Design review of the part built by this model. Coordinates are the model's own, in mm. Give positions to 0.01 mm unless a question says otherwise; leave off trailing zeros. Loops run counter-clockwise (first coordinate to the right, second up) from the corner with the lowest first, then second, coordinate; pieces in that order, holes last. Notation, with made-up numbers: M 89,-36 L 144,-36 A29 ccw 144,-8 Z; hole C 37,25 d5. An arc over 180 degrees is marked long. Use a Markdown table: item, result. Add a question column.
(1) Add section A-A, the plane y = 0. Give the boundary of the cut face in (x, z), then the cut area to 3 significant figures.
(2) Add section C-C, the plane z = -10. Give the boundary of the cut face in (x, y), then the cut area to 3 significant figures.
(3) For probe 1 along Z at (x, y) = (1.25, 0); probe 2 along Z at (x, y) = (1.55, -1.75); probe 3 along Y at (x, z) = (1.4, -16), list the stretches that pass through material, from the lowest coordinate up.
(4) Draft analysis for pull direction Y (two halves, no side actions). For faces 1 (the face through (1, 0, 19.5)), 2 (the face through (1, 0, 17)), 3 (the face through (0.9, -11, 0.3)), state which applies: pulls with the +Y half, pulls with the -Y half, needs draft (parallel to the pull), parting line crosses it, or undercut.
(5) Add section B-B, the plane z = -15. Give the boundary of the cut face in (x, y), then the cut area to 3 significant figures.
```python
from build123d import *

# Parameters (mm, degrees)
PAD011_DEPTH       = 19.5
SKETCH016_R        = 2
POCKET003_DEPTH    = 2.3
CHAMFER006_1_SIZE2 = 4
CHAMFER006_1_SIZE  = 1.5
CHAMFER006_2_SIZE2 = 4
CHAMFER006_2_SIZE  = 1.5
CHAMFER007_SIZE    = 0.2


with BuildPart() as part:
    # Sketch015 → Pad011 (new body, symmetric)
    with BuildSketch(Plane.XY):
        Polygon((0, -10.1), (0, 10.1), (1.8, 11.9), (2.3, 11.9), (2.3, -11.9), (1.8, -11.9), align=None)
    extrude(amount=PAD011_DEPTH, both=True)

    # Sketch016 (on Face4 of Pad011) → Pocket003 (cut)
    with BuildSketch(Plane.YZ.offset(2.3)):
        with Locations((0, 15)):
            Circle(SKETCH016_R)
        with Locations((0, -15)):
            Circle(SKETCH016_R)
    extrude(amount=-POCKET003_DEPTH, mode=Mode.SUBTRACT)

    # Chamfer006 1
    chamfer006_1_edges = [part.edges().sort_by_distance(p)[0] for p in [
        (2.05, -11.9, -19.5),
        (2.05, 11.9, -19.5),
    ]]
    chamfer006_1_side = part.faces().sort_by_distance((1.184602, 0, -19.5))[0]
    chamfer(chamfer006_1_edges, length=CHAMFER006_1_SIZE, length2=CHAMFER006_1_SIZE2, reference=chamfer006_1_side)

    # Chamfer006 2
    chamfer006_2_edges = [part.edges().sort_by_distance(p)[0] for p in [
        (2.05, -11.9, 19.5),
        (2.05, 11.9, 19.5),
    ]]
    chamfer006_2_side = part.faces().sort_by_distance((1.184602, 0, 19.5))[0]
    chamfer(chamfer006_2_edges, length=CHAMFER006_2_SIZE, length2=CHAMFER006_2_SIZE2, reference=chamfer006_2_side)

    # Chamfer007
    chamfer007_edges = [part.edges().sort_by_distance(p)[0] for p in [
        (2.3, -2, -15),
        (0, -2, -15),
        (2.3, -2, 15),
        (0, -2, 15),
    ]]
    chamfer(chamfer007_edges, length=CHAMFER007_SIZE)


solid = part.part
```
Established:
| question | item | result |
|---|---|---|
| 1 | outline | M 0,-19.5 L 2.3,-19.5 L 2.3,-17.2 L 2.1,-17 L 0.2,-17 L 0,-17.2 Z; M 0,-12.8 L 0.2,-13 L 2.1,-13 L 2.3,-12.8 L 2.3,12.8 L 2.1,13 L 0.2,13 L 0,12.8 Z; M 0,17.2 L 0.2,17 L 2.1,17 L 2.3,17.2 L 2.3,19.5 L 0,19.5 Z |
| 1 | area | 71.1 mm^2 |
| 2 | outline | M 0,-10.1 L 1.8,-11.9 L 2.3,-11.9 L 2.3,11.9 L 1.8,11.9 L 0,10.1 Z |
| 2 | area | 51.5 mm^2 |
| 3 | probe 1 | -19.5 to -17, -13 to 13, 17 to 19.5 |
| 3 | probe 2 | -19.5 to -15.97, -14.03 to 14.03, 15.97 to 19.5 |
| 3 | probe 3 | -11.5 to -1.73, 1.73 to 11.5 |
| 4 | face 1 | needs draft |
| 4 | face 2 | undercut |
| 4 | face 3 | pulls with the -Y half |
| 5 | outline | M 0,-10.1 L 1.8,-11.9 L 2.3,-11.9 L 2.3,-2.2 L 2.1,-2 L 0.2,-2 L 0,-2.2 Z; M 0,2.2 L 0.2,2 L 2.1,2 L 2.3,2.2 L 2.3,11.9 L 1.8,11.9 L 0,10.1 Z |
| 5 | area | 42.2 mm^2 |
